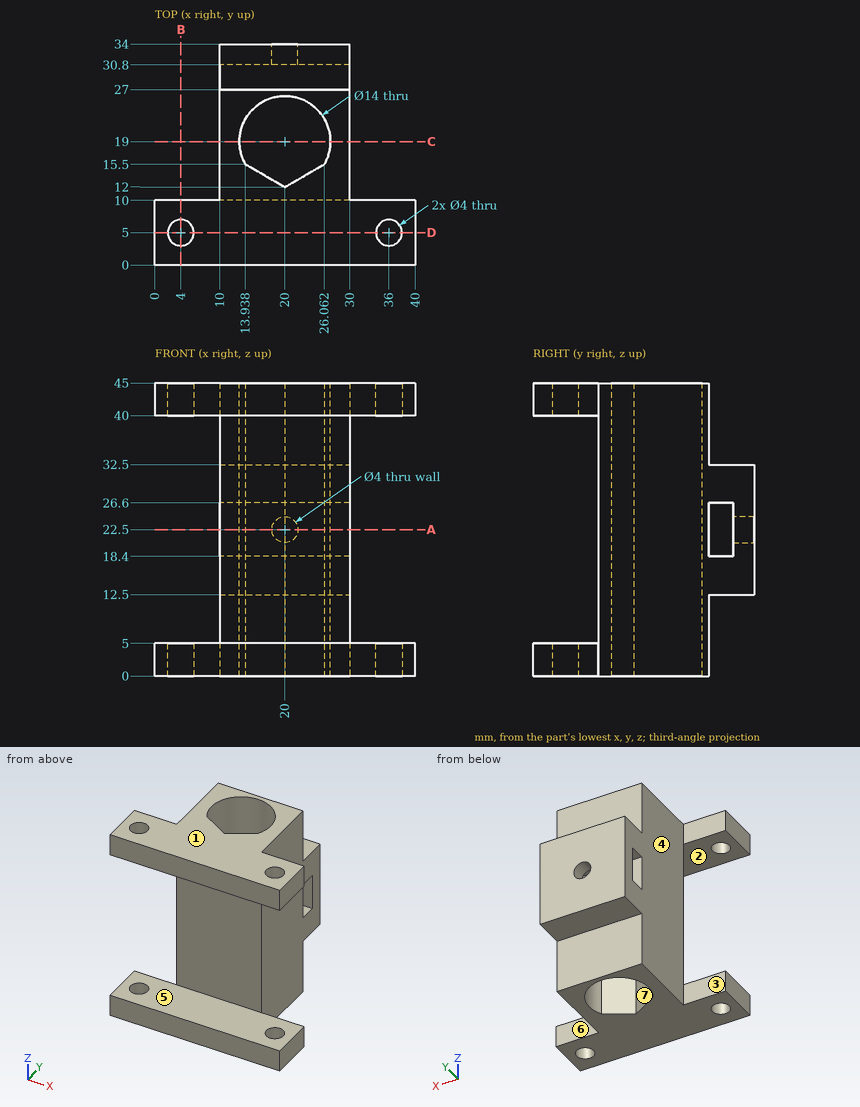
The figure shows three views and two pictorial views of one solid part (mm, origin at its lowest corner). Answer the questions. A direction names the side the tool comes from. Round coordinates to 2 decimals unless told otherwise and drop trailing zeros. Write each loop counter-clockwise with the first axis right and the second up, starting at its lowest first coordinate (ties: lowest second). Pieces come first, ordered by that corner, then holes. Notation, with made-up numbers: M -30.75,81 L -4.75,81 A21 cw -4.75,88 Z; hole C 50,74.5 d8. An arc over 180 degrees is marked long. Write each question's results on one line, items separated by ' | '. Start each with the question number.
(1) Each of these flat-tipped pins is pushed along its axis until it touches: P1, Ø6.5, axis at x = 36, y = 5, coming from the -Z side; P2, Ø5, axis at y = 10.5, z = 24, coming from the -X side; P3, Ø3, axis at x = 19, z = 17.5, coming from the -Y side; P4, Ø2.5, axis at x = 33.5, z = 2.5, coming from the +Y side. Where does it stop, or does it pass through?
(2) The part is cut by section A-A, the plane z = 22.5. Write down the section's boundary in (x, y), and give its area (3 significant figures).
(3) The part is cut by section B-B, the plane x = 4. Write down the section's boundary in (y, z), and give its area (3 significant figures).
(4) Find the intervals of material crossed by line 1 (Y direction, x = 4, z = 1); line 2 (X direction, y = 31.6, z = 22.5); line 3 (X direction, y = 4, z = 41), in increasing order.
(5) Determine the mould class of the marked faces 1, 2 and 3 for opening direction Z: +Z half, -Z half, draft (parallel to the pull), parting line (faces both ways), or undercut.
(6) For the marked faces 4, 5, 6 and 7, determine the directions among +Z, -Z, +X, -X, +Y, -Y from which every point of the face is accessible in a straight line to the end or side of a thin tool.
(7) The part is cut by section D-D, the plane y = 5. Write down the section's boundary in (x, z).
(8) The part is cut by section C-C, the plane y = 19. Write down the section's boundary in (x, z), and give its area (3 significant figures).
Worked answers:
1) P1: stops at z = 0 | P2: stops at x = 10 | P3: stops at y = 10 | P4: stops at y = 10
2) outline: M 10,10 L 30,10 L 30,27 L 10,27 Z; M 10,30.8 L 18,30.8 L 18,34 L 10,34 Z; M 22,30.8 L 30,30.8 L 30,34 L 22,34 Z; hole M 13.94,15.5 L 20,12 L 26.06,15.5 A7 ccw long Z | area: 246 mm²
3) outline: M 0,0 L 3,0 L 3,5 L 0,5 Z; M 0,40 L 3,40 L 3,45 L 0,45 Z; M 7,0 L 10,0 L 10,5 L 7,5 Z; M 7,40 L 10,40 L 10,45 L 7,45 Z | area: 60.0 mm²
4) line 1: y = 0 to 3, 7 to 10 | line 2: x = 10 to 18, 22 to 30 | line 3: x = 0 to 2.27, 5.73 to 34.27, 37.73 to 40
5) face 1: +Z half | face 2: undercut | face 3: draft
6) face 4: +Z, -Z, -X, +Y | face 5: +X, -X, -Y | face 6: +Z, -Z, +X, +Y | face 7: +Z, -Z
7) outline: M 0,0 L 2,0 L 2,5 L 0,5 Z; M 0,40 L 2,40 L 2,45 L 0,45 Z; M 6,0 L 34,0 L 34,5 L 6,5 Z; M 6,40 L 34,40 L 34,45 L 6,45 Z; M 38,0 L 40,0 L 40,5 L 38,5 Z; M 38,40 L 40,40 L 40,45 L 38,45 Z
8) outline: M 10,0 L 13,0 L 13,45 L 10,45 Z; M 27,0 L 30,0 L 30,45 L 27,45 Z | area: 270 mm²
